from build123d import *

# Parameters (mm, degrees)
F2_R = 0.5
F3_R = 0.5


with BuildPart() as f1:
    # F0 (on Front) → F1 (revolve)
    with BuildSketch(Plane.XZ):
        Polygon((8, 4.2), (0, 4.2), (0, 0), (5.3, 0), (8, 3.809567), align=None)
    revolve(axis=Axis((0, 0, 2.1), (0, 0, 1)))

    # F2
    f2_edges = [f1.edges().sort_by_distance(p)[0] for p in [
        (-5.3, 0, 0),
    ]]
    fillet(f2_edges, radius=F2_R)

    # F3
    f3_edges = [f1.edges().sort_by_distance(p)[0] for p in [
        (-8, 0, 3.809567),
    ]]
    fillet(f3_edges, radius=F3_R)


solid = f1.part
Part model, mm, in its own coordinate system. Coordinates: 2 decimals unless noted, no trailing zeros. Loops run counter-clockwise (first coordinate to the right, second up) from the corner with the lowest first, then second, coordinate; pieces in that order, holes last. Notation, with made-up numbers: (31.5, 56.25) -> (43.5, 56.25) arc R11 ccw to (43.5, 68.25) -> close; hole circle Ø1 at (89, 43). An arc over 180 degrees is marked (long way). Use a Markdown table: item, result. Add a question column.
Item 1: Flat gauge pins, fed straight in: P1, Ø2, axis at x = -2, y = 2.5, coming from the -Z side; P2, Ø2, axis at x = -5.5, z = 2, coming from the -Y side. Where does each tip first touch, or does it go through?
Item 2: Probe probe 1 along Y at (x, z) = (1.75, 0.6); probe 2 along Z at (x, y) = (-2, 7.25); probe 3 along X at (y, z) = (-2, 1.2). List the from-to ranges inside material, lowest first.
Item 3: Band-saw the part on A-A on z = 0.6. Write the cut outline in (x, y).
Item 4: Band-saw the part on B-B on z = 2.35. Write the cut outline in (x, y), plus the area to 3 significant figures.
Geometry says:
| question | item | result |
|---|---|---|
| 1 | P1 | z = 0 |
| 1 | P2 | y = -5.4 |
| 2 | probe 1 | -5.45 to 5.45 |
| 2 | probe 2 | 3.13 to 4.2 |
| 2 | probe 3 | -5.82 to 5.82 |
| 3 | outline | circle Ø11.45 at (0, 0) |
| 4 | outline | circle Ø13.93 at (0, 0) |
| 4 | area | 152 mm² |
